```python
from build123d import *

# Parameters (mm, degrees)
BOSS_EXTRUDE1_DEPTH = 16.5
CHAMFER1_SIZE       = 6
FILLET1_R           = 10


with BuildPart() as part:
    # Sketch1 → Boss-Extrude1 (new, symmetric)
    with BuildSketch(Plane.XY):
        Polygon((15.875, 0), (9.6, 0), (9.6, 12.9), (-9.6, 12.9), (-9.6, 0), (-15.875, 0), (-15.875, 19.05), (15.875, 19.05), align=None)
    extrude(amount=BOSS_EXTRUDE1_DEPTH, both=True)

    # Chamfer1
    chamfer1_edges = [part.edges().sort_by_distance(p)[0] for p in [
        (15.875, 9.525, 16.5),
        (0, 19.05, 16.5),
        (-15.875, 9.525, 16.5),
    ]]
    chamfer(chamfer1_edges, length=CHAMFER1_SIZE)

    # Fillet1
    fillet1_edges = [part.edges().sort_by_distance(p)[0] for p in [
        (-15.875, 19.05, -3),
        (15.875, 19.05, -3),
    ]]
    fillet(fillet1_edges, radius=FILLET1_R)


solid = part.part
```
Input: part model. Units: mm. Frame: model coordinates. A direction names the side the tool comes from. Give positions to 0.01 mm unless a question says otherwise; leave off trailing zeros. Order: outer loops, then holes, each group sorted by start corner. A loop starts at its lowest first (then second) coordinate and runs counter-clockwise, first axis right, second up. Notation, with made-up numbers: (75, 52) - (125, 52) arc R14 ccw to (125, 58) - close; hole circle Ø9 at (-24.5, 18). An arc over 180 degrees is marked (long way). Put each result on its own line as item: value.
Item 1: Section query B-B, the plane z = -11. Return loops of the section in (x, y) (3 decimals), then the cut area to 3 significant figures.
Found:
outline: (-15.875, 0) - (-9.6, 0) - (-9.6, 12.9) - (9.6, 12.9) - (9.6, 0) - (15.875, 0) - (15.875, 9.05) arc R10 ccw to (5.875, 19.05) - (-5.875, 19.05) arc R10 ccw to (-15.875, 9.05) - close
area: 314 mm^2
Item 2: Access query for faces 1 (the cylindrical face through (13.023, 16.043, -1.326)), 2 (the flat face through (-9.6, 7, 0)). Directions: +Z, -Z, +X, -X, +Y, -Y. A direction counts if a zero-diameter tool reaches every point of the face in a straight line with its end or side. Return the directions, or none.
Found:
face 1: +Z, -Z, +X, +Y
face 2: +Z, -Z, -Y
Item 3: Draft query along Z for faces 3 (the flat face through (0, 14, -16.5)), 4 (the flat face through (-12.917, 7.948, 13.458)), 5 (the cylindrical face through (-12.868, 16.198, -1.326)). Return one class per face: +Z half, -Z half, draft (parallel to the pull), parting line (faces both ways), or undercut.
Found:
face 3: -Z half
face 4: +Z half
face 5: draft
Item 4: Section query A-A, the plane y = 3.5. Return loops of the section in (x, z) (3 decimals).
Found:
outline: (-15.875, -16.5) - (-9.6, -16.5) - (-9.6, 16.5) - (-9.875, 16.5) - (-15.875, 10.5) - close; (9.6, -16.5) - (15.875, -16.5) - (15.875, 10.5) - (9.875, 16.5) - (9.6, 16.5) - close
Item 5: Contact query for flat-ended pins moving along their axis: pin 1 (10 mm diameter, centred on x = 11, y = 4.5, fed in from +Z); pin 2 (4 mm diameter, centred on x = 12.5, z = 11.5, fed in from +Y); pin 3 (6 mm diameter, centred on x = 2, z = -8, fed in from -Y). Output: stop coordinate, or through.
Found:
pin 1: stops at z = 16.5
pin 2: stops at y = 17.92
pin 3: stops at y = 12.9
Item 6: Section query C-C, the plane x = -1. Return loops of the section in (y, z).
Found:
outline: (12.9, -16.5) - (19.05, -16.5) - (19.05, 10.5) - (13.05, 16.5) - (12.9, 16.5) - close
Item 7: Ray query, L1, parallel to X at y = 3.25, z = -6 (3 decimals); L2, parallel to Y at x = 5, z = 3; L3, parallel to X at y = 1, z = 12.5 (3 decimals). Return the intervals inside material, ascending. Write a range as from..to.
Found:
L1: x = -15.875..-9.6, 9.6..15.875
L2: y = 12.9..19.05
L3: x = -13.875..-9.6, 9.6..13.875
Item 8: Section query D-D, the plane y = 10.75. Return loops of the section in (x, z) (3 decimals), then the cut area to 3 significant figures.
Found:
outline: (-15.729, -16.5) - (-9.6, -16.5) - (-9.6, 16.5) - (-9.875, 16.5) - (-15.729, 10.646) - close; (9.6, -16.5) - (15.729, -16.5) - (15.729, 10.646) - (9.875, 16.5) - (9.6, 16.5) - close
area: 370 mm^2
